```python
from build123d import *

# Parameters (mm, degrees)
SKETCH009_R     = 1.75
PAD004_DEPTH    = 2
SKETCH010_W     = 15
SKETCH010_H     = 5
PAD005_DEPTH    = 10
POCKET005_DEPTH = 5
SKETCH012_R     = 1.75
POCKET006_DEPTH = 5
FILLET003_R     = 2


with BuildPart() as part:
    # Sketch009 → Pad004 (new body)
    with BuildSketch(Plane.XY):
        with BuildLine():
            ThreePointArc((0, -12), (3, -9), (0, -6))
            Line((-4.999996, -6), (0, -6))
            ThreePointArc((-5.000003, 6), (-11, -3e-06), (-4.999996, -6))
            Line((-5.000003, 6), (0, 6))
            ThreePointArc((0, 6), (3, 9), (0, 12))
            Line((-5.000044, 12), (0, 12))
            ThreePointArc((-5.000044, 12), (-17, -2.2e-05), (-5, -12))
            Line((0, -12), (-5, -12))
        make_face()
        with Locations((0, -9)):
            Circle(SKETCH009_R, mode=Mode.SUBTRACT)
        with Locations((0, 9)):
            Circle(SKETCH009_R, mode=Mode.SUBTRACT)
    extrude(amount=PAD004_DEPTH)

    # Sketch010 → Pad005 (join)
    with BuildSketch(Plane.XY):
        with Locations((-19.5, 0)):
            Rectangle(SKETCH010_W, SKETCH010_H)
    extrude(amount=PAD005_DEPTH)

    # Sketch011 (on Face16 of Pad005) → Pocket005 (cut)
    with BuildSketch(Plane.XZ.offset(2.5)):
        Polygon((-12, 2), (-20, 10), (-12, 10), align=None)
    extrude(amount=-POCKET005_DEPTH, mode=Mode.SUBTRACT)

    # Sketch012 (on Face17 of Pocket005) → Pocket006 (cut)
    with BuildSketch(Plane.XZ.offset(2.5)):
        with Locations((-23, 5)):
            Circle(SKETCH012_R)
    extrude(amount=-POCKET006_DEPTH, mode=Mode.SUBTRACT)

    # Fillet003
    fillet003_edges = [part.edges().sort_by_distance(p)[0] for p in [
        (-12, 0, 2),
        (-14.368347, 2.5, 2),
        (-14.368347, -2.5, 2),
        (-16.736695, -2.5, 1),
        (-16.736695, 2.5, 1),
    ]]
    fillet(fillet003_edges, radius=FILLET003_R)


solid = part.part
```
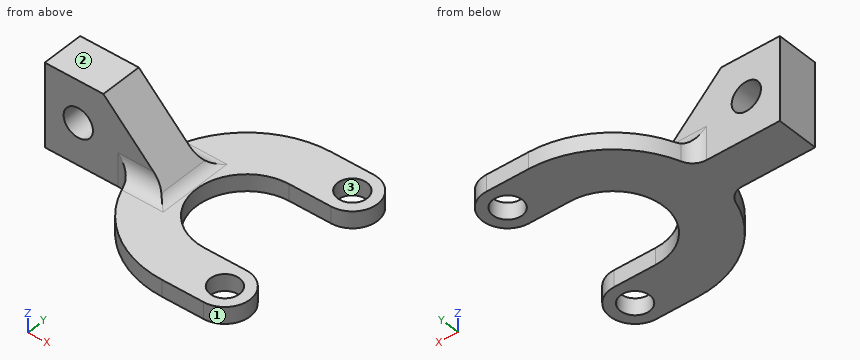
Can you work these out from the model? Positions are in its coordinate system, mm. Face numbers are marked on the shaded views. Round coordinates to 2 decimals unless told otherwise and drop trailing zeros. Loops run counter-clockwise (first coordinate to the right, second up) from the corner with the lowest first, then second, coordinate; pieces in that order, holes last.
Item 1: Suppose I cut it at C-C, the plane x = -3. Write out the boundary of the cut face in (y, z).
Item 2: Suppose I cut it at D-D, the plane y = -9. Write out the boundary of the cut face in (x, z).
Item 3: If we mould it in two halves opening along X, with no side actions, what happens to the marked faces 1, 2 and 3? For each: +X half, -X half, draft (parallel to the pull), parting line (faces both ways), or undercut.
Item 4: Will these pins go through, and if not, where does the flat tip stop? pin 1 Ø5 at (x, y) = (-23.5, -1.5) entering from -Z; pin 2 Ø1.5 at (x, z) = (-19.5, 3.5) entering from +Y; pin 3 Ø1 at (y, z) = (-5.5, 4) entering from +X; pin 4 Ø5.5 at (x, y) = (-7, -6) entering from +Z.
Item 5: Please list where these lines run through material, in increasing order: L1, parallel to Y at x = 0, z = 1.15; L2, parallel to Y at x = -5.25, z = 1.5; L3, parallel to Z at x = -23, y = 0.45.
Item 6: Suppose I cut it at B-B, the plane z = 1.5. Write out the boundary of the cut face in (x, y).
Item 7: Suppose I cut it at A-A, the plane y = 0. Write out the boundary of the cut face in (x, z), then the cut area to 3 significant figures.
Reported:
1. outline: (-12, 0) - (-6, 0) - (-6, 2) - (-12, 2) - close; (6, 0) - (12, 0) - (12, 2) - (6, 2) - close
2. outline: (-12.94, 0) - (-1.75, 0) - (-1.75, 2) - (-12.94, 2) - close; (1.75, 0) - (3, 0) - (3, 2) - (1.75, 2) - close
3. face 1: +X half
3. face 2: draft
3. face 3: undercut
4. pin 1: stops at z = 0
4. pin 2: stops at y = 2.5
4. pin 3: passes through
4. pin 4: stops at z = 2
5. L1: y = -12 to -10.75, -7.25 to -6, 6 to 7.25, 10.75 to 12
5. L2: y = -12 to -5.99, 5.99 to 12
5. L3: z = 0 to 3.25, 6.75 to 10
6. outline: (-27, -2.5) - (-18.26, -2.5) arc R2 cw to (-16.36, -3.86) arc R12 ccw to (-5, -12) - (0, -12) arc R3 ccw to (0, -6) - (-5, -6) arc R6 cw to (-5, 6) - (0, 6) arc R3 ccw to (0, 12) - (-5, 12) arc R12 ccw to (-16.36, 3.86) arc R2 cw to (-18.26, 2.5) - (-27, 2.5) - close; hole circle Ø3.5 at (0, -9); hole circle Ø3.5 at (0, 9)
7. outline: (-27, 0) - (-11, 0) - (-11, 2) - (-11.17, 2) arc R2 cw to (-12.59, 2.59) - (-20, 10) - (-27, 10) - close; hole circle Ø3.5 at (-23, 5)
7. area: 110 mm2
